Geometry: final body of the model. Coordinates: model frame, mm. A direction names the side the tool comes from. Coordinates: 2 decimals unless noted, no trailing zeros. Write each loop counter-clockwise with the first axis right and the second up, starting at its lowest first coordinate (ties: lowest second). Pieces come first, ordered by that corner, then holes. Notation, with made-up numbers: (22.5, 28.25) - (79.5, 28.25) arc R26 ccw to (79.5, 58.25) - close; hole circle Ø10 at (-21.5, -0.75). An arc over 180 degrees is marked (long way). Answer as a JSON object with one key per item and string values. Group by question number.
Item 1: Section A-A on x = -6. Return loops of the section in (y, z), and give its area (3 significant figures).
Item 2: Set-up query: faces 5 (the cylindrical face through (14.01, -6.99, 47.15)), 6 (the flat face through (-10.6, -8, 26)), 7 (the cylindrical face through (-10, -9, 26)). Return all of +Z, -Z, +X, -X, +Y, -Y with unobstructed straight access to the full face (end or side cutting, diameter ignored); none if empty.
Item 3: First-contact query: pin 1 Ø4 at (x, y) = (10.5, 2.5) entering from +Z; pin 2 Ø11 at (x, z) = (-1.5, 27.5) entering from -Y; pin 3 Ø1.5 at (x, y) = (-3, -5) entering from +Z. Flat tips, straight axial feed; report the tip coordinate or a pass-through.
Item 4: Section B-B on z = 32.5. Return loops of the section in (x, y), and give its area (3 significant figures).
Item 5: Mould query, pull axis X, two halves, no side actions, for faces 1 (the flat face through (15, 0, 25)), 2 (the flat face through (0, 8, 27)), 3 (the flat face through (0, 0, 0)), 4 (the cylindrical face through (-12.43, -7.4, 26.06)). Classes: pulls with the +X half, pulls with the -X half, needs draft (parallel to the pull), parting line crosses it, or undercut.
Item 6: Section C-C on y = 3. Return loops of the section in (x, z), and give its area (3 significant figures).
Item 7: Section D-D on x = 12. Return loops of the section in (y, z).
Item 8: Line query: line 1 along X through (y, z) = (6, 42); line 2 along Z through (x, y) = (-3, 4.25); line 3 along Y through (x, z) = (-4.25, 43.5). Output: solid intervals per line, ascending. Write a range as from..to.
```python
from build123d import *

# Parameters (mm, degrees)
F0_W     = 30
F0_H     = 20
F0_W_2   = 26
F0_H_2   = 16
F1_DEPTH = 50
F2_W     = 30
F2_H     = 20
F3_DEPTH = 2
F5_DEPTH = 2
F6_R     = 10
F7_R     = 2


with BuildPart() as f1:
    # F0 (on Top) → F1 (new body)
    with BuildSketch(Plane.XY):
        Rectangle(F0_W, F0_H)
        Rectangle(F0_W_2, F0_H_2, mode=Mode.SUBTRACT)
    extrude(amount=F1_DEPTH)

    # F2 (on Top) → F3 (join)
    with BuildSketch(Plane.XY):
        Rectangle(F2_W, F2_H)
    extrude(amount=F3_DEPTH)

    # F4 (on face) → F5 (cut, through all)
    with BuildSketch(Plane.XZ.offset(10)):
        with BuildLine():
            Line((13, 50), (-13, 50))
            Line((-13, 50), (-13, 30.582575695))
            ThreePointArc((-13, 30.582575695), (-10, 26), (-13, 21.417424305))
            Line((-13, 21.417424305), (-13, 2))
            Line((-13, 2), (-4.582575695, 2))
            ThreePointArc((-4.582575695, 2), (0, 5), (4.582575695, 2))
            Line((4.582575695, 2), (13, 2))
            Line((13, 2), (13, 21.417424305))
            ThreePointArc((13, 21.417424305), (10, 26), (13, 30.582575695))
            Line((13, 30.582575695), (13, 50))
        make_face()
    extrude(amount=-F5_DEPTH, mode=Mode.SUBTRACT)

    # F6
    f6_edges = [f1.edges().sort_by_distance(p)[0] for p in [
        (14, -10, 50),
        (-14, -10, 50),
    ]]
    fillet(f6_edges, radius=F6_R)

    # F7
    f7_edges = [f1.edges().sort_by_distance(p)[0] for p in [
        (13, -1, 2),
        (13, 8, 26),
        (0, 8, 2),
        (-13, -1, 2),
        (-13, 8, 26),
        (13, -8, 26),
        (-13, -8, 26),
        (0, -8, 2),
    ]]
    fillet(f7_edges, radius=F7_R)


solid = f1.part
```
Checks:
{
 "1": {"outline": "(-10, 0) - (10, 0) - (10, 50) - (8, 50) - (8, 4) arc R2 cw to (6, 2) - (-10, 2) - close", "area": "137 mm^2"},
 "2": {"face 5": "+Z, +X, -X, -Y", "face 6": "+Z", "face 7": "-Y"},
 "3": {"pin 1": "z = 2.68", "pin 2": "y = 8", "pin 3": "z = 2"},
 "4": {"outline": "(-15, -10) - (-13, -10) - (-13, 6) arc R2 cw to (-11, 8) - (11, 8) arc R2 cw to (13, 6) - (13, -10) - (15, -10) - (15, 10) - (-15, 10) - close", "area": "134 mm^2"},
 "5": {"face 1": "pulls with the +X half", "face 2": "undercut", "face 3": "needs draft", "face 4": "undercut"},
 "6": {"outline": "(-15, 0) - (15, 0) - (15, 50) - (13, 50) - (13, 4) arc R2 cw to (11, 2) - (-11, 2) arc R2 cw to (-13, 4) - (-13, 50) - (-15, 50) - close", "area": "254 mm^2"},
 "7": {"outline": "(-10, 0) - (10, 0) - (10, 50) - (7.73, 50) - (7.73, 4) arc R1.73 cw to (6, 2.27) - (-10, 2.27) - close; (-10, 22) - (-7.73, 22) - (-7.73, 30) - (-10, 30) - close"},
 "8": {"line 1": "-15..-13, 13..15", "line 2": "0..2", "line 3": "8..10"}
}
